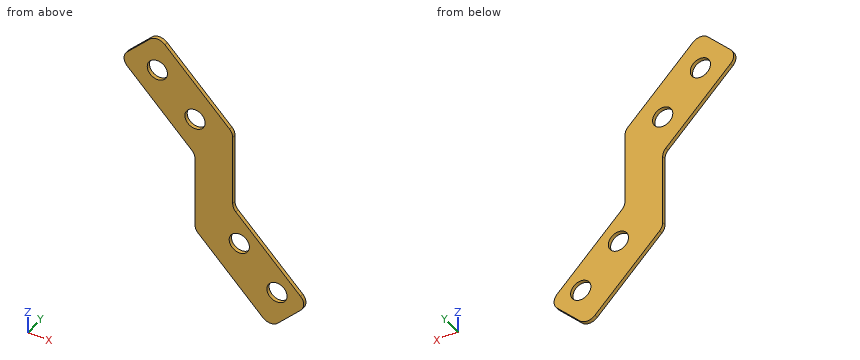
from build123d import *

# Parameters (mm, degrees)
BASE_FLANGE2_DEPTH    = 0.7
F_6_CLEARANCE_HOLE1_D = 3.7973
FILLET1_R             = 2


# Sheet-metal steps are written as plain solids
with BuildPart() as part:
    # Sketch1 → Base-Flange2 (new body)
    with BuildSketch(Plane(origin=(0, 0, 0), x_dir=(1, 0, 0), z_dir=(0, 1, 0))):
        Polygon((0, 0), (0, 15), (14.142135624, 29.142135624), (7.071067812, 36.213203436), (-7.071067812, 22.071067812), (-7.071067812, 7.071067812), (-21.213203436, -7.071067812), (-14.142135624, -14.142135624), align=None)
    extrude(amount=-BASE_FLANGE2_DEPTH)

    # #6 Clearance Hole1 (through all)
    with Locations(Plane(origin=(0, 0, 0), x_dir=(1, 0, 0), z_dir=(0, 1, 0))):
        with Locations((-14.139821541, -7.073381895), (-7.068753729, -0.002314083), (1.237436867, 21.653874811), (8.308504679, 28.724942623)):
            Hole(F_6_CLEARANCE_HOLE1_D / 2)

    # Fillet1
    fillet1_edges = [part.edges().sort_by_distance(p)[0] for p in [
        (-14.142135624, -0.35, 14.142135624),
        (-21.213203436, -0.35, 7.071067812),
        (-7.071067812, -0.35, -7.071067812),
        (-7.071067812, -0.35, -22.071067812),
        (7.071067812, -0.35, -36.213203436),
        (14.142135624, -0.35, -29.142135624),
        (0, -0.35, -15),
        (0, -0.35, 0),
    ]]
    fillet(fillet1_edges, radius=FILLET1_R)


solid = part.part
Design review of the part built by this model. Coordinates are the model's own, in mm. Give positions to 0.01 mm unless a question says otherwise; leave off trailing zeros. Order: outer loops, then holes, each group sorted by start corner. A loop starts at its lowest first (then second) coordinate and runs counter-clockwise, first axis right, second up. Notation, with made-up numbers: (10, 45.25) - (33, 45.25) arc R37 ccw to (33, 82.25) - close; hole circle Ø11 at (46.25, 19). An arc over 180 degrees is marked (long way). Use CSV: the item, a comma, the result in double quotes. Start each with the question number.
Q1. Take a section at C-C (x = -2.5). State the section outline as (y, z) points, and give its area (3 significant figures).
Q2. Take a section at A-A (y = -0.4). State the section outline as (x, z) points.
Q3. For line 1 (Z direction, x = 2, y = -0.4); line 2 (X direction, y = -0.05, z = -8.5); line 3 (Z direction, x = 8, y = -0.25), list the stretches that pass through material, from the lowest coordinate up.
Q4. Take a section at B-B (z = -17). State the section outline as (x, y) points, and give its area (3 significant figures).
Q5. For P1, Ø5, axis at x = -7.07, z = 0, coming from the -Y side, flat-tipped, find the tip position at first contact; note if it passes through.
Calculated:
1,outline,"(-0.7, -26.64) - (0, -26.64) - (0, 2.5) - (-0.7, 2.5) - close"
1,area,"20.4 mm²"
2,outline,"(-19.8, 5.66) - (-7.66, -6.49) arc R2 cw to (-7.07, -7.9) - (-7.07, -21.24) arc R2 ccw to (-6.49, -22.66) - (5.66, -34.8) arc R2 ccw to (8.49, -34.8) - (12.73, -30.56) arc R2 ccw to (12.73, -27.73) - (0.59, -15.59) arc R2 cw to (0, -14.17) - (0, -0.83) arc R2 ccw to (-0.59, 0.59) - (-12.73, 12.73) arc R2 ccw to (-15.56, 12.73) - (-19.8, 8.49) arc R2 ccw to start; hole circle Ø3.8 at (-14.14, 7.07); hole circle Ø3.8 at (-7.07, 0); hole circle Ø3.8 at (1.24, -21.65); hole circle Ø3.8 at (8.31, -28.72)"
3,line 1,"z = -31.14 to -23.39, -19.92 to -17"
3,line 2,"x = -7.07 to 0"
3,line 3,"z = -35.16 to -30.6, -26.85 to -23"
4,outline,"(-7.07, -0.7) - (2, -0.7) - (2, 0) - (-7.07, 0) - close"
4,area,"6.35 mm²"
5,P1,"stops at y = -0.7"
